from build123d import *

# Parameters (mm, degrees)
RESSALTO_EXTRUS_O1_DEPTH = 2.5
ESBO_O2_W                = 30.81
ESBO_O2_H                = 3
RESSALTO_EXTRUS_O2_DEPTH = 9.5
ESBO_O3_W                = 17.8
ESBO_O3_H                = 1
CORTE_EXTRUS_O1_DEPTH    = 10
ESBO_O4_W                = 30.81
ESBO_O4_H                = 1.5
RESSALTO_EXTRUS_O3_DEPTH = 1
ESBO_O5_W                = 17.8
ESBO_O5_H                = 9.5
RESSALTO_EXTRUS_O4_DEPTH = 9.5
FILETE1_R                = 1.5
CORTE_EXTRUS_O2_DEPTH    = 22.715524976
ESBO_O7_W                = 3.5
ESBO_O7_H                = 4.25
CORTE_EXTRUS_O3_DEPTH    = 2
ESBO_O8_W                = 3.5
ESBO_O8_H                = 6.727306506
CORTE_EXTRUS_O4_DEPTH    = 1.5
ESBO_O9_R                = 1.35
CORTE_EXTRUS_O5_DEPTH    = 21.503085743
ESBO_O10_W               = 0.8
ESBO_O10_H               = 2
CORTE_EXTRUS_O6_DEPTH    = 2.5
PADR_O_LINEAR1_COUNT     = 3
PADR_O_LINEAR1_PITCH     = 2.77
PADR_O_LINEAR1_COL_COUNT = 3
PADR_O_LINEAR1_COL_PITCH = 2.77
ESBO_O11_W               = 0.8
ESBO_O11_H               = 4.7
CORTE_EXTRUS_O7_DEPTH    = 1
ESBO_O12_W               = 0.8
ESBO_O12_H               = 1.5
CORTE_EXTRUS_O8_DEPTH    = 2
PADR_O_LINEAR2_COUNT     = 4
PADR_O_LINEAR2_PITCH     = 2.77


with BuildPart() as part:
    # Esboço1 → Ressalto-extrusão1 (new body)
    with BuildSketch(Plane.XY):
        with BuildLine():
            Line((-13.405, 6.25), (13.405, 6.25))
            ThreePointArc((13.405, 6.25), (14.819213562, 5.664213562), (15.405, 4.25))
            Line((15.405, 4.25), (15.405, -6.25))
            Line((15.405, -6.25), (-15.405, -6.25))
            Line((-15.405, -6.25), (-15.405, 4.25))
            ThreePointArc((-15.405, 4.25), (-14.819213562, 5.664213562), (-13.405, 6.25))
        make_face()
    extrude(amount=-RESSALTO_EXTRUS_O1_DEPTH)

    # Esboço2 → Ressalto-extrusão2 (add)
    with BuildSketch(Plane(origin=(0, 0, -2.5), x_dir=(-1, 0, 0), z_dir=(0, 0, -1))):
        with Locations((0, -4.75)):
            Rectangle(ESBO_O2_W, ESBO_O2_H)
    extrude(amount=RESSALTO_EXTRUS_O2_DEPTH)

    # Esboço3 → Corte-extrusão1 (cut)
    with BuildSketch(Plane(origin=(0, 0, -12), x_dir=(-1, 0, 0), z_dir=(0, 0, -1))):
        with Locations((0, -5.75)):
            Rectangle(ESBO_O3_W, ESBO_O3_H)
    extrude(amount=-CORTE_EXTRUS_O1_DEPTH, mode=Mode.SUBTRACT)

    # Esboço4 → Ressalto-extrusão3 (add)
    with BuildSketch(Plane(origin=(0, 0, -2.5), x_dir=(-1, 0, 0), z_dir=(0, 0, -1))):
        with Locations((0, 3.5)):
            Rectangle(ESBO_O4_W, ESBO_O4_H)
    extrude(amount=RESSALTO_EXTRUS_O3_DEPTH)

    # Esboço5 → Ressalto-extrusão4 (add)
    with BuildSketch(Plane(origin=(0, 0, -2.5), x_dir=(-1, 0, 0), z_dir=(0, 0, -1))):
        with Locations((0, -0.5)):
            Rectangle(ESBO_O5_W, ESBO_O5_H)
    extrude(amount=RESSALTO_EXTRUS_O4_DEPTH)

    # Filete1
    filete1_edges = [part.edges().sort_by_distance(p)[0] for p in [
        (8.9, 4.25, -7.75),
        (-8.9, 4.25, -7.75),
    ]]
    fillet(filete1_edges, radius=FILETE1_R)

    # Esboço6 → Corte-extrusão2 (cut, through all)
    with BuildSketch(Plane(origin=(0, -3.25, 0), x_dir=(1, 0, 0), z_dir=(0, 1, 0))):
        with BuildLine():
            Line((10.745, 6.25), (10.745, 9.25))
            ThreePointArc((10.745, 9.25), (12.495, 11), (14.245, 9.25))
            Line((14.245, 9.25), (14.245, 6.25))
            ThreePointArc((14.245, 6.25), (12.495, 4.5), (10.745, 6.25))
        make_face()
    corte_extrus_o2 = extrude(amount=-CORTE_EXTRUS_O2_DEPTH, mode=Mode.SUBTRACT)

    # Espelhar1: Corte-extrusão2 across plane
    add(corte_extrus_o2.mirror(Plane(origin=(0, 0, 0), x_dir=(0, 0, 1), z_dir=(1, 0, 0))), mode=Mode.SUBTRACT)

    # Esboço7 → Corte-extrusão3 (cut)
    with BuildSketch(Plane(origin=(0, -3.25, 0), x_dir=(1, 0, 0), z_dir=(0, 1, 0))):
        with Locations((12.495, 9.875)):
            Rectangle(ESBO_O7_W, ESBO_O7_H)
    corte_extrus_o3 = extrude(amount=-CORTE_EXTRUS_O3_DEPTH, mode=Mode.SUBTRACT)

    # Espelhar2: Corte-extrusão3 across plane
    add(corte_extrus_o3.mirror(Plane(origin=(0, 0, 0), x_dir=(0, 0, 1), z_dir=(1, 0, 0))), mode=Mode.SUBTRACT)

    # Esboço8 → Corte-extrusão4 (cut)
    with BuildSketch(Plane.XZ.offset(6.25)):
        with Locations((-12.495, -3.363653253)):
            Rectangle(ESBO_O8_W, ESBO_O8_H)
    corte_extrus_o4 = extrude(amount=-CORTE_EXTRUS_O4_DEPTH, mode=Mode.SUBTRACT)

    # Espelhar3: Corte-extrusão3, Corte-extrusão4 across plane
    add(corte_extrus_o3.mirror(Plane(origin=(0, 0, 0), x_dir=(0, 0, 1), z_dir=(1, 0, 0))), mode=Mode.SUBTRACT)
    add(corte_extrus_o4.mirror(Plane(origin=(0, 0, 0), x_dir=(0, 0, 1), z_dir=(1, 0, 0))), mode=Mode.SUBTRACT)

    # Esboço9 → Corte-extrusão5 (cut, through all)
    with BuildSketch(Plane.XY):
        with Locations((12.495, 0)):
            Circle(ESBO_O9_R)
    corte_extrus_o5 = extrude(amount=-CORTE_EXTRUS_O5_DEPTH, mode=Mode.SUBTRACT)

    # Espelhar4: Corte-extrusão5 across plane
    add(corte_extrus_o5.mirror(Plane(origin=(0, 0, 0), x_dir=(0, 0, 1), z_dir=(1, 0, 0))), mode=Mode.SUBTRACT)

    # Esboço10 → Corte-extrusão6 (cut)
    with BuildSketch(Plane.XZ.offset(5.25)):
        with Locations((0, -11)):
            Rectangle(ESBO_O10_W, ESBO_O10_H)
    corte_extrus_o6 = extrude(amount=-CORTE_EXTRUS_O6_DEPTH, mode=Mode.SUBTRACT)

    # Padrão linear1: Corte-extrusão6 ×3
    with Locations(*[(-i * PADR_O_LINEAR1_PITCH, 0, 0) for i in range(1, PADR_O_LINEAR1_COUNT)]):
        add(corte_extrus_o6, mode=Mode.SUBTRACT)

    # Padrão linear1 col: Corte-extrusão6 ×3
    with Locations(*[(i * PADR_O_LINEAR1_COL_PITCH, 0, 0) for i in range(1, PADR_O_LINEAR1_COL_COUNT)]):
        add(corte_extrus_o6, mode=Mode.SUBTRACT)

    # Esboço11 → Corte-extrusão7 (cut)
    with BuildSketch(Plane.XZ.offset(5.25)):
        with Locations((4.155, -9.65)):
            Rectangle(ESBO_O11_W, ESBO_O11_H)
    corte_extrus_o7 = extrude(amount=-CORTE_EXTRUS_O7_DEPTH, mode=Mode.SUBTRACT)

    # Esboço12 → Corte-extrusão8 (cut)
    with BuildSketch(Plane(origin=(0, 0, -12), x_dir=(-1, 0, 0), z_dir=(0, 0, -1))):
        with Locations((-4.155, -3.5)):
            Rectangle(ESBO_O12_W, ESBO_O12_H)
    corte_extrus_o8 = extrude(amount=-CORTE_EXTRUS_O8_DEPTH, mode=Mode.SUBTRACT)

    # Padrão linear2: Corte-extrusão7, Corte-extrusão8 ×4
    with Locations(*[(-i * PADR_O_LINEAR2_PITCH, 0, 0) for i in range(1, PADR_O_LINEAR2_COUNT)]):
        add(corte_extrus_o7, mode=Mode.SUBTRACT)
        add(corte_extrus_o8, mode=Mode.SUBTRACT)


solid = part.part
Build history of the part. All positions in model axes, mm. A direction names the side the tool comes from. Round coordinates to 2 decimals unless told otherwise and drop trailing zeros. Loops run counter-clockwise (first coordinate to the right, second up) from the corner with the lowest first, then second, coordinate; pieces in that order, holes last. Notation, with made-up numbers: (71, 8.5) -> (123, 8.5) arc R15 cw to (123, 18.5) -> close; hole circle Ø4 at (64, 64.25). An arc over 180 degrees is marked (long way). One line per item, written item: value. Start each with the question number.
Q1. Cut at C-C on y = 2. List the corners of the cut face in (x, z) (3 decimals).
Q2. Cut at D-D on z = -0.75. List the corners of the cut face in (x, y) (3 decimals), plus the area to 3 significant figures.
Q3. Cut at A-A on z = -3. List the corners of the cut face in (x, y) (3 decimals).
Q4. Cut at B-B on x = 1.5. List the corners of the cut face in (y, z).
Q5. Drop flat-ended pins along their axis: pin 1 Ø5 at (x, z) = (-12, -8) entering from +Y; pin 2 Ø2 at (y, z) = (2, -8) entering from +X; pin 3 Ø0.6 at (x, z) = (-4, -10.5) entering from -Y. Give the stop position or say it passes through.
Q6. 3-axis set-ups, long thin cutter, end or side, ignore diameter. For faces 5 (the face through (0, -6, -2)), 6 (the face through (-13.78, 0.41, -1.23)), 7 (the face through (0, -6.25, -1)), 8 (the face through (-12, 4, -3.5)), 9 (the face through (-10.745, -5, -7)): which of +Z, -Z, +X, -X, +Y, -Y reach the whole face in a straight line?
Q7. Two-plate mould, pull along Y, no slides. Class faces 1 (the face through (12, 2.75, -3)), 2 (the face through (-12, 2.75, -3)), 3 (the face through (0.985, -4.3, -10.2)), 4 (the face through (4, -4.25, -9)): released by +Y, released by -Y, zero draft, split by the parting line, or undercut.
Q8. Probe line 1 along Y through (x, z) = (9, -11); line 2 along Y through (x, z) = (0, -7); line 3 along Z through (x, y) = (-14, 2). List the from-to ranges inside material, lowest first.
Computed:
1. outline: (-15.405, -2.5) -> (-8.9, -2.5) -> (-8.9, -12) -> (8.9, -12) -> (8.9, -2.5) -> (15.405, -2.5) -> (15.405, 0) -> (-15.405, 0) -> close
2. outline: (-15.405, -6.25) -> (-14.245, -6.25) -> (-14.245, -4.75) -> (-10.745, -4.75) -> (-10.745, -6.25) -> (10.745, -6.25) -> (10.745, -4.75) -> (14.245, -4.75) -> (14.245, -6.25) -> (15.405, -6.25) -> (15.405, 4.25) arc R2 ccw to (13.405, 6.25) -> (-13.405, 6.25) arc R2 ccw to (-15.405, 4.25) -> close; hole circle Ø2.7 at (-12.495, 0); hole circle Ø2.7 at (12.495, 0)
2. area: 361 mm²
3. outline: (-15.405, -6.25) -> (-14.245, -6.25) -> (-14.245, -4.75) -> (-10.745, -4.75) -> (-10.745, -6.25) -> (-8.9, -6.25) -> (-8.9, -5.25) -> (8.9, -5.25) -> (8.9, -6.25) -> (10.745, -6.25) -> (10.745, -4.75) -> (14.245, -4.75) -> (14.245, -6.25) -> (15.405, -6.25) -> (15.405, -3.25) -> (8.9, -3.25) -> (8.9, 2.75) -> (15.405, 2.75) -> (15.405, 4.25) -> (-15.405, 4.25) -> (-15.405, 2.75) -> (-8.9, 2.75) -> (-8.9, -3.25) -> (-15.405, -3.25) -> close
4. outline: (-6.25, -2) -> (-5.25, -2) -> (-5.25, -7.3) -> (-4.25, -7.3) -> (-4.25, -10) -> (-2.75, -10) -> (-2.75, -12) -> (4.25, -12) -> (4.25, -2.5) -> (6.25, -2.5) -> (6.25, 0) -> (-6.25, 0) -> close
5. pin 1: y = -3.25
5. pin 2: x = 8.9
5. pin 3: y = -5.25
6. face 5: -Z, -Y
6. face 6: +Z, -Z
6. face 7: +Z, -Z, +X, -X, -Y
6. face 8: -Z, -X, +Y
6. face 9: none
7. face 1: undercut
7. face 2: undercut
7. face 3: zero draft
7. face 4: released by -Y
8. line 1: -6.25 to -3.25
8. line 2: -5.25 to 4.25
8. line 3: -2.5 to 0
